Can you work these out from the model? Positions are in its coordinate system, mm. A direction names the side the tool comes from. Give positions to 0.01 mm unless a question says otherwise; leave off trailing zeros. Answer as a JSON object with one key per item and string values.
```python
from build123d import *

# Parameters (mm, degrees)
SKETCH1_W               = 50.8
SKETCH1_H               = 314.489898324
BOSS_EXTRUDE1_DEPTH     = 25.4
CUT_EXTRUDE1_DEPTH      = 162.295672716
SKETCH3_R               = 3.175
CUT_EXTRUDE2_DEPTH      = 162.295672716
SKETCH6_W               = 25.4
SKETCH6_H               = 50.8
BOSS_EXTRUDE3_DEPTH     = 152.4
CUT_EXTRUDE4_DEPTH      = 312.721533651
CUT_EXTRUDE5_DEPTH      = 315.810728123
SKETCH5_R               = 2.38125
CUT_EXTRUDE3_DEPTH      = 312.543594923
CUT_EXTRUDE6_DEPTH      = 469.269684217
CUT_EXTRUDE6_DEPTH_BACK = 152.4
SKETCH9_R               = 29.953527753
SKETCH9_W               = 20.828
SKETCH9_H               = 33.528


with BuildPart() as part:
    # Sketch1 → Boss-Extrude1 (new body)
    with BuildSketch(Plane(origin=(0, 0, 0), x_dir=(0, 0, -1), z_dir=(1, 0, 0))):
        Rectangle(SKETCH1_W, SKETCH1_H)
    extrude(amount=BOSS_EXTRUDE1_DEPTH)

    # Sketch2 → Cut-Extrude1 (cut, through all)
    with BuildSketch(Plane(origin=(25.4, 0, 0), x_dir=(0, 0, -1), z_dir=(1, 0, 0))):
        Polygon((-25.4, -157.244949162), (25.4, -121.674406221), (50.8, -121.674406221), (50.8, -172.474406221), (-25.4, -172.474406221), align=None)
    extrude(amount=-CUT_EXTRUDE1_DEPTH, mode=Mode.SUBTRACT)

    # Sketch3 → Cut-Extrude2 (cut, through all)
    with BuildSketch(Plane(origin=(25.4, 0, 0), x_dir=(0, 0, -1), z_dir=(1, 0, 0))):
        with Locations((-13.004038703, -133.061366341)):
            Circle(SKETCH3_R)
        with Locations((13.004038703, -114.850314487)):
            Circle(SKETCH3_R)
        with Locations((0, 81.044949162)):
            Circle(SKETCH3_R)
    extrude(amount=-CUT_EXTRUDE2_DEPTH, mode=Mode.SUBTRACT)

    # Sketch6 → Boss-Extrude3 (add)
    with BuildSketch(Plane(origin=(0, 157.244949162, 0), x_dir=(1, 0, 0), z_dir=(0, 1, 0))):
        with Locations((12.7, 0)):
            Rectangle(SKETCH6_W, SKETCH6_H)
    extrude(amount=BOSS_EXTRUDE3_DEPTH)

    # Sketch7 → Cut-Extrude4 (cut, through all)
    with BuildSketch(Plane(origin=(25.4, 0, 0), x_dir=(0, 0, -1), z_dir=(1, 0, 0))):
        with BuildLine():
            Line((-25.4, 157.244949162), (-25.4, 309.644949162))
            Line((-25.4, 309.644949162), (-13.97, 309.644949162))
            Line((-13.97, 309.644949162), (-13.97, 163.594949162))
            ThreePointArc((-13.97, 163.594949162), (-15.829871939, 159.104821101), (-20.32, 157.244949162))
            Line((-20.32, 157.244949162), (-25.4, 157.244949162))
        make_face()
        with BuildLine():
            Line((39.293979998, 157.244949162), (25.908, 157.244949162))
            ThreePointArc((25.908, 157.244949162), (21.417871939, 159.104821101), (19.558, 163.594949162))
            Line((19.558, 163.594949162), (19.558, 309.644949162))
            Line((19.558, 309.644949162), (39.293979998, 309.644949162))
            Line((39.293979998, 309.644949162), (39.293979998, 157.244949162))
        make_face()
    extrude(amount=-CUT_EXTRUDE4_DEPTH, mode=Mode.SUBTRACT)

    # Sketch8 → Cut-Extrude5 (cut, through all)
    with BuildSketch(Plane.XY.offset(25.4)):
        with BuildLine():
            Line((2.286, 309.644949162), (-14.90160116, 309.644949162))
            Line((-14.90160116, 309.644949162), (-14.90160116, 157.244949162))
            Line((-14.90160116, 157.244949162), (-4.064, 157.244949162))
            ThreePointArc((-4.064, 157.244949162), (0.426128061, 159.104821101), (2.286, 163.594949162))
            Line((2.286, 163.594949162), (2.286, 309.644949162))
        make_face()
        with BuildLine():
            Line((23.114, 163.594949162), (23.114, 309.644949162))
            Line((23.114, 309.644949162), (40.983283112, 309.644949162))
            Line((40.983283112, 309.644949162), (40.983283112, 157.244949162))
            Line((40.983283112, 157.244949162), (29.464, 157.244949162))
            ThreePointArc((29.464, 157.244949162), (24.973871939, 159.104821101), (23.114, 163.594949162))
        make_face()
    extrude(amount=-CUT_EXTRUDE5_DEPTH, mode=Mode.SUBTRACT)

    # Sketch5 → Cut-Extrude3 (cut, through all)
    with BuildSketch(Plane(origin=(23.114, 0, 0), x_dir=(0, 0, -1), z_dir=(1, 0, 0))):
        with Locations(Location((2.794, 296.956244864, 0), (0, 0, 90))):
            Circle(SKETCH5_R)
        with Locations(Location((2.794, 176.306244864, 0), (0, 0, 90))):
            Circle(SKETCH5_R)
    extrude(amount=-CUT_EXTRUDE3_DEPTH, mode=Mode.SUBTRACT)

    # Sketch9 → Cut-Extrude6 (cut, two sides: drawn at the far end of the back side and taken through both)
    # profile 1 of 3: a face of its own
    with BuildSketch(Plane(origin=(0, 309.644949162, 0), x_dir=(1, 0, 0), z_dir=(0, 1, 0)).offset(-CUT_EXTRUDE6_DEPTH_BACK)):
        with Locations((12.7, 2.794)):
            Circle(SKETCH9_R)
        with Locations((12.7, 2.794)):
            Rectangle(SKETCH9_W, SKETCH9_H, mode=Mode.SUBTRACT)
    # profile 2 of 3: a face of its own
    with BuildSketch(Plane(origin=(0, 309.644949162, 0), x_dir=(1, 0, 0), z_dir=(0, 1, 0)).offset(-CUT_EXTRUDE6_DEPTH_BACK)):
        Polygon((3.302, 18.542), (12.7, 18.542), (12.7, 19.558), (2.286, 19.558), (2.286, -13.97), (12.7, -13.97), (12.7, -12.954), (3.302, -12.954), align=None)
    # profile 3 of 3: a face of its own
    with BuildSketch(Plane(origin=(0, 309.644949162, 0), x_dir=(1, 0, 0), z_dir=(0, 1, 0)).offset(-CUT_EXTRUDE6_DEPTH_BACK)):
        Polygon((12.7, 18.542), (22.098, 18.542), (22.098, 2.794), (22.098, -12.954), (12.7, -12.954), (12.7, -13.97), (23.114, -13.97), (23.114, 19.558), (12.7, 19.558), align=None)
    extrude(amount=CUT_EXTRUDE6_DEPTH + CUT_EXTRUDE6_DEPTH_BACK, mode=Mode.SUBTRACT)


solid = part.part
```
1) I'm going to push flat-ended pins straight in: P1, Ø4, axis at y = 296.96, z = -2.79, coming from the -X side; P2, Ø9.5, axis at y = 224, z = -1.5, coming from the -X side; P3, Ø9.5, axis at x = 12, y = 227, coming from the +Z side; P4, Ø9.5, axis at x = 12, y = 268.5, coming from the -Z side. Where does each tip first touch, or does it pass through?
Check sheet entries:
{"P1": "through", "P2": "x = 3.3", "P3": "z = 12.95", "P4": "z = -18.54"}
2) Imagine slicing it at A-A on x = 13.5. Give the number of separate pieces and of enclosed holes in the cut face, and give its area (3 significant figures).
Check sheet entries:
{"separate pieces": "1", "enclosed holes": "5", "area": "19,700 mm2"}
3) Which directions (+Z, -Z, +X, -X, +Y, -Y) give clear straight access to the entire face, cutting with the end or side of a thin tool? Please do faces 1 (the flat face through (22.098, 232, -3)), 2 (the flat face through (13, 232, -18.542)), 3 (the flat face through (13, 232, 12.954)), 4 (the flat face through (3.302, 232, -3)).
Check sheet entries:
{"face 1": "+Z, -Z, +X, +Y", "face 2": "-Z, +X, -X, +Y", "face 3": "+Z, +X, -X, +Y", "face 4": "+Z, -Z, -X, +Y"}
4) I need wall thicknesses on L1, parallel to Z at x = 11.25, y = 246; L2, parallel to X at y = 169, z = 8.5; L3, parallel to Y at x = 13.25, z = 0. Which ranges of each line are inside material? Lowest first, please.
Check sheet entries:
{"L1": "-18.54 to 12.95", "L2": "3.3 to 22.1", "L3": "-139.46 to 77.87, 84.22 to 309.64"}
